```python
from build123d import *

# Parameters (mm, degrees)
SKETCH_1_R   = 4.765
SKETCH_1_R_2 = 3.58


with BuildPart() as part:
    # По траектории1: sweep along a curve in space
    with BuildLine() as sweep_1_path:
        Line((0, 0, 0), (0, 0, 15))
        ThreePointArc((0, 0, 15), (0.060917298, 0, 18.48994967), (0.243594974, 0, 21.975647374))
        Line((0.243594974, 0, 21.975647374), (3.033853924, 0, 61.878209385))
    # Эскиз1 → По траектории1 (sweep)
    with BuildSketch(Plane.XY):
        Circle(SKETCH_1_R)
        Circle(SKETCH_1_R_2, mode=Mode.SUBTRACT)
    sweep(path=sweep_1_path.line)


solid = part.part
```
Geometry: final body of the model. Coordinates: model frame, mm. Round coordinates to 2 decimals unless told otherwise and drop trailing zeros. Loops run counter-clockwise (first coordinate to the right, second up) from the corner with the lowest first, then second, coordinate; pieces in that order, holes last.
Item 1: Line query: L1, parallel to Y at x = 0, z = 7 (3 decimals); L2, parallel to X at y = -0.25, z = 10; L3, parallel to Y at x = 1.25, z = 58.5. Output: solid intervals per line, ascending.
Checked values:
L1: y = -4.765 to -3.58, 3.58 to 4.765
L2: x = -4.76 to -3.57, 3.57 to 4.76
L3: y = -4.51 to -3.23, 3.23 to 4.51
Item 2: Mould query, pull axis Y, two halves, no side actions, for faces 1 (the cylindrical face through (-0.776, -3.495, 7.605)), 2 (the flat face through (1, 4, 0)), 3 (the cylindrical face through (-0.62, 4.724, 7.605)). Classes: released by +Y, released by -Y, zero draft, split by the parting line, or undercut.
Checked values:
face 1: undercut
face 2: zero draft
face 3: split by the parting line
Item 3: Section A-A, the plane y = 0. Output: boundary loops of the cut face in (x, z) (3 decimals), plus the area to 3 significant figures.
Checked values:
outline: (-4.765, 0) - (-3.58, 0) - (-3.58, 15) arc R103.58 cw to (-3.328, 22.225) - (-0.537, 62.128) - (-1.72, 62.211) - (-4.51, 22.308) arc R104.765 ccw to (-4.765, 15) - close; (3.58, 0) - (4.765, 0) - (4.765, 15) arc R95.235 cw to (4.997, 21.643) - (7.787, 61.546) - (6.605, 61.628) - (3.815, 21.726) arc R96.42 ccw to (3.58, 15) - close
area: 147 mm2
Item 4: Contact query for flat-ended pins moving along their axis: P1, Ø1, axis at x = 6, z = 47.5, coming from the -Y side; P2, Ø2, axis at y = 2.5, z = 33, coming from the +X side; P3, Ø2, axis at y = -2, z = 12, coming from the +X side; P4, Ø1.5, axis at x = 2, y = 0, coming from the -Z side. Output: stop coordinate, or through.
Checked values:
P1: stops at y = -3.27
P2: stops at x = 5.56
P3: stops at x = 4.66
P4: passes through
Item 5: Section B-B, the plane y = -2.75. Output: boundary loops of the cut face in (x, z), plus the area to 3 significant figures.
Checked values:
outline: (-3.89, 0) - (-2.29, 0) - (-2.29, 15) arc R102.29 cw to (-2.04, 22.14) - (0.75, 62.04) - (-0.85, 62.15) - (-3.64, 22.25) arc R103.89 ccw to (-3.89, 15) - close; (2.29, 0) - (3.89, 0) - (3.89, 15) arc R96.11 cw to (4.13, 21.7) - (6.92, 61.61) - (5.32, 61.72) - (2.53, 21.82) arc R97.71 ccw to (2.29, 15) - close
area: 198 mm2
